Input: part model. Units: mm. Frame: model coordinates. A direction names the side the tool comes from. Coordinates: 2 decimals unless noted, no trailing zeros. Loops run counter-clockwise (first coordinate to the right, second up) from the corner with the lowest first, then second, coordinate; pieces in that order, holes last. Notation, with made-up numbers: (-24, 45.25) -> (-10, 45.25) arc R10 ccw to (-10, 51.25) -> close; hole circle Ø10 at (-19.5, 11.25). An arc over 180 degrees is marked (long way). Put each result on its own line as item: value. Start each with the question number.
1) Cut plane A-A (z = -80). Return the cut outline in (x, y), plus the area to 3 significant figures.
2) Cut plane D-D (y = 2.45). State how many separate pieces and enclosed holes the cut face has, plus the area to 3 significant figures.
3) Contact query for flat-ended pins moving along their axis: P1, Ø1, axis at y = 2, z = -71.5, coming from the -X side; P2, Ø3, axis at x = 38, z = -87.5, coming from the -Y side. Output: stop coordinate, or through.
4) Cut plane B-B (x = 17). Return the cut outline in (y, z), plus the area to 3 significant figures.
5) Set-up query: faces 4 (the flat face through (20, 2, -60)), 5 (the flat face through (65, 2, -12)), 6 (the flat face through (42, 3, -42)). Return all of +Z, -Z, +X, -X, +Y, -Y with unobstructed straight access to the full face (end or side cutting, diameter ignored); none if empty.
6) Pull-direction query (Z, two-part tool) for faces 1 (the cylindrical face through (84, 2, -104)), 2 (the cylindrical face through (15.5, 1.52, -10.07)), 3 (the flat face through (0, 1, -30)); classes: pulls with the +Z half, pulls with the -Z half, needs draft (parallel to the pull), parting line crosses it, or undercut.
7) Material intervals for L1, parallel to X at y = 2.55, z = -43; L2, parallel to X at y = 1.1, z = -46.8; L3, parallel to Z at x = 72.5, y = 2.15, sorted ascending.
8) Cut plane C-C (x = 55.5). Return the cut outline in (y, z).
from build123d import *

# Parameters (mm, degrees)
SKETCH1_W           = 86
SKETCH1_H           = 105
BOSS_EXTRUDE1_DEPTH = 3
SKETCH2_W           = 3
SKETCH2_H           = 5
CUT_EXTRUDE1_DEPTH  = 3
LPATTERN1_COUNT     = 3
LPATTERN1_PITCH     = 30
SKETCH5_R           = 1.5
CUT_EXTRUDE2_DEPTH  = 4
SKETCH6_R           = 3
SKETCH6_W           = 11
SKETCH6_H           = 55
CUT_EXTRUDE3_DEPTH  = 4
FILLET2_R           = 2
SKETCH7_W           = 41
SKETCH7_H           = 45
CUT_EXTRUDE4_DEPTH  = 4
FILLET3_R           = 5


with BuildPart() as part:
    # Sketch1 → Boss-Extrude1 (new body)
    with BuildSketch(Plane(origin=(0, 0, 0), x_dir=(1, 0, 0), z_dir=(0, 1, 0))):
        with Locations((43, 52.5)):
            Rectangle(SKETCH1_W, SKETCH1_H)
    extrude(amount=BOSS_EXTRUDE1_DEPTH)

    # Sketch2 → Cut-Extrude1 (cut)
    with BuildSketch(Plane(origin=(0, 3, 0), x_dir=(1, 0, 0), z_dir=(0, 1, 0))):
        with Locations((63.5, 12.5)):
            Rectangle(SKETCH2_W, SKETCH2_H)
        with Locations((47.5, 12.5)):
            Rectangle(SKETCH2_W, SKETCH2_H)
        with Locations((27.5, 12.5)):
            Rectangle(SKETCH2_W, SKETCH2_H)
        with Locations((6.5, 12.5)):
            Rectangle(SKETCH2_W, SKETCH2_H)
        with Locations((81.3, 12.5)):
            Rectangle(SKETCH2_W, SKETCH2_H)
    cut_extrude1 = extrude(amount=-CUT_EXTRUDE1_DEPTH, mode=Mode.SUBTRACT)

    # LPattern1: Cut-Extrude1 ×3
    with Locations(*[(0, 0, -i * LPATTERN1_PITCH) for i in range(1, LPATTERN1_COUNT)]):
        add(cut_extrude1, mode=Mode.SUBTRACT)

    # Sketch5 → Cut-Extrude2 (cut, through all)
    with BuildSketch(Plane(origin=(0, 3, 0), x_dir=(1, 0, 0), z_dir=(0, 1, 0))):
        with Locations((17, 10)):
            Circle(SKETCH5_R)
        with Locations((17, 50)):
            Circle(SKETCH5_R)
        with Locations((72.5, 10)):
            Circle(SKETCH5_R)
        with Locations((55.5, 90)):
            Circle(SKETCH5_R)
    extrude(amount=-CUT_EXTRUDE2_DEPTH, mode=Mode.SUBTRACT)

    # Sketch6 → Cut-Extrude3 (cut, through all)
    with BuildSketch(Plane(origin=(0, 3, 0), x_dir=(1, 0, 0), z_dir=(0, 1, 0))):
        with Locations((34, 11.8)):
            Circle(SKETCH6_R)
        with Locations((34, 46.8)):
            Circle(SKETCH6_R)
        with Locations((74.3, 65)):
            Rectangle(SKETCH6_W, SKETCH6_H)
    extrude(amount=-CUT_EXTRUDE3_DEPTH, mode=Mode.SUBTRACT)

    # Fillet2
    fillet2_edges = [part.edges().sort_by_distance(p)[0] for p in [
        (79.8, 1.5, -92.5),
        (68.8, 1.5, -37.5),
        (68.8, 1.5, -92.5),
        (79.8, 1.5, -37.5),
    ]]
    fillet(fillet2_edges, radius=FILLET2_R)

    # Sketch7 → Cut-Extrude4 (cut, through all)
    with BuildSketch(Plane(origin=(0, 3, 0), x_dir=(1, 0, 0), z_dir=(0, 1, 0))):
        with Locations((20.5, 82.5)):
            Rectangle(SKETCH7_W, SKETCH7_H)
    extrude(amount=-CUT_EXTRUDE4_DEPTH, mode=Mode.SUBTRACT)

    # Fillet3
    fillet3_edges = [part.edges().sort_by_distance(p)[0] for p in [
        (0, 1.5, -60),
        (41, 1.5, -105),
        (41, 1.5, -60),
        (86, 1.5, -105),
        (86, 1.5, 0),
        (0, 1.5, 0),
    ]]
    fillet(fillet3_edges, radius=FILLET3_R)


solid = part.part
Results found:
1. outline: (41, 0) -> (68.8, 0) -> (68.8, 3) -> (41, 3) -> close; (79.8, 0) -> (86, 0) -> (86, 3) -> (79.8, 3) -> close
1. area: 102 mm2
2. separate pieces: 1
2. enclosed holes: 18
2. area: 6,280 mm2
3. P1: stops at x = 41
3. P2: passes through
4. outline: (0, -60) -> (3, -60) -> (3, -51.5) -> (0, -51.5) -> close; (0, -48.5) -> (3, -48.5) -> (3, -11.5) -> (0, -11.5) -> close; (0, -8.5) -> (3, -8.5) -> (3, 0) -> (0, 0) -> close
4. area: 162 mm2
5. face 4: -Z, -X, +Y, -Y
5. face 5: +Y, -Y
5. face 6: +Z, -Z, +X, -X, +Y
6. face 1: pulls with the -Z half
6. face 2: undercut
6. face 3: needs draft
7. L1: x = 0 to 5, 8 to 26, 29 to 46, 49 to 62, 65 to 68.8, 82.8 to 86
7. L2: x = 0 to 31, 37 to 68.8, 79.8 to 86
7. L3: z = -105 to -92.5, -37.5 to -11.5, -8.5 to 0
8. outline: (0, -105) -> (3, -105) -> (3, -91.5) -> (0, -91.5) -> close; (0, -88.5) -> (3, -88.5) -> (3, 0) -> (0, 0) -> close
